```python
from build123d import *

# Parameters (mm, degrees)
SKETCH1_W           = 130
SKETCH1_H           = 98.5
SKETCH1_R           = 36.5
SKETCH1_R_2         = 5
BOSS_EXTRUDE1_DEPTH = 6
SKETCH2_W           = 130
SKETCH2_H           = 6
BOSS_EXTRUDE2_DEPTH = 75
CHAMFER1_SIZE       = 8
CUT_EXTRUDE1_DEPTH  = 7
BOSS_EXTRUDE3_START = -0.1
BOSS_EXTRUDE3_DEPTH = 3
BOSS_EXTRUDE4_START = -0.1
BOSS_EXTRUDE4_DEPTH = 3
FILLET1_R           = 2


with BuildPart() as part:
    # Sketch1 → Boss-Extrude1 (new body)
    with BuildSketch(Plane.XY):
        with Locations((-0.4, 43.207953426)):
            Rectangle(SKETCH1_W, SKETCH1_H)
        with Locations((-0.4, 45.807953426)):
            Circle(SKETCH1_R, mode=Mode.SUBTRACT)
        with Locations((-35.2, 80.607953426)):
            Circle(SKETCH1_R_2, mode=Mode.SUBTRACT)
        with Locations((34.4, 80.607953426)):
            Circle(SKETCH1_R_2, mode=Mode.SUBTRACT)
        with Locations((34.4, 11.007953426)):
            Circle(SKETCH1_R_2, mode=Mode.SUBTRACT)
        with Locations((-35.2, 11.007953426)):
            Circle(SKETCH1_R_2, mode=Mode.SUBTRACT)
    extrude(amount=BOSS_EXTRUDE1_DEPTH)

    # Sketch2 → Boss-Extrude2 (add)
    with BuildSketch(Plane.XY.offset(6)):
        with Locations((-0.4, -3.042046574)):
            Rectangle(SKETCH2_W, SKETCH2_H)
    extrude(amount=BOSS_EXTRUDE2_DEPTH)

    # Chamfer1
    chamfer1_edges = [part.edges().sort_by_distance(p)[0] for p in [
        (-65.4, -3.042046574, 81),
        (64.6, -3.042046574, 81),
        (-65.4, 92.457953426, 3),
        (64.6, 92.457953426, 3),
    ]]
    chamfer(chamfer1_edges, length=CHAMFER1_SIZE)

    # Sketch3 → Cut-Extrude1 (cut, through all)
    with BuildSketch(Plane(origin=(0, -0.042046574, 0), x_dir=(1, 0, 0), z_dir=(0, 1, 0))):
        with BuildLine():
            Line((-58.9, -68.5), (-58.9, -18.5))
            ThreePointArc((-58.9, -18.5), (-55.4, -15), (-51.9, -18.5))
            Line((-51.9, -18.5), (-51.9, -68.5))
            ThreePointArc((-51.9, -68.5), (-55.4, -72), (-58.9, -68.5))
        make_face()
        with BuildLine():
            Line((58.1, -68.5), (58.1, -18.5))
            ThreePointArc((58.1, -18.5), (54.6, -15), (51.1, -18.5))
            Line((51.1, -18.5), (51.1, -68.5))
            ThreePointArc((51.1, -68.5), (54.6, -72), (58.1, -68.5))
        make_face()
    extrude(amount=-CUT_EXTRUDE1_DEPTH, mode=Mode.SUBTRACT)

    # Sketch4 → Boss-Extrude3 (add)
    with BuildSketch(Plane.ZY.offset(65.4).offset(BOSS_EXTRUDE3_START)):
        Polygon((6, 37.957953426), (35, -0.042046574), (12.357101974, -0.042046574), (6, 8.287949116), align=None)
    extrude(amount=-BOSS_EXTRUDE3_DEPTH)

    # Sketch5 → Boss-Extrude4 (add)
    with BuildSketch(Plane(origin=(64.6, 0, 0), x_dir=(0, 0, -1), z_dir=(1, 0, 0)).offset(BOSS_EXTRUDE4_START)):
        Polygon((-6, 8.287949116), (-6, 37.957953426), (-35, -0.042046574), (-12.357101974, -0.042046574), align=None)
    extrude(amount=-BOSS_EXTRUDE4_DEPTH)

    # Fillet1
    fillet1_edges = [part.edges().sort_by_distance(p)[0] for p in [
        (-0.4, -0.042046574, 6),
        (-0.4, -6.042046574, 0),
    ]]
    fillet(fillet1_edges, radius=FILLET1_R)


solid = part.part
```
For this review, take the finished solid that the model builds, in its own axes (mm). A direction names the side the tool comes from. Round coordinates to 2 decimals unless told otherwise and drop trailing zeros. Order: outer loops, then holes, each group sorted by start corner. A loop starts at its lowest first (then second) coordinate and runs counter-clockwise, first axis right, second up.
Q1. We need section D-D, the plane x = -0.4. Give the boundary of the cut face in (y, z), plus the area to 3 significant figures.
Findings below:
outline: (-6.04, 2) arc R2 ccw to (-4.04, 0) - (9.31, 0) - (9.31, 6) - (1.96, 6) arc R2 cw to (-0.04, 8) - (-0.04, 81) - (-6.04, 81) - close; (82.31, 0) - (92.46, 0) - (92.46, 6) - (82.31, 6) - close
area: 603 mm2
Q2. Insertion check: P1, Ø2, axis at x = 20, z = 59, coming from the +Y side; P2, Ø6, axis at x = -51.5, y = 51, coming from the +Z side; P3, Ø8, axis at x = -27, y = 75.5, coming from the -Z side; P4, Ø14.5, axis at y = 10, z = 18, coming from the -X side. Each pin has a flat end and moves straight along its axis. Give the tip position at first contact, or say it passes through.
Findings below:
P1: stops at y = -0.04
P2: stops at z = 6
P3: stops at z = 0
P4: stops at x = -65.3
Q3. Wall thickness on line 1 (X direction, y = -0.5, z = 53); line 2 (Y direction, x = -0.4, z = 1.8); line 3 (X direction, y = 12.5, z = 21): over which ranges is each line inside the solid? List them lowest first.
Findings below:
line 1: x = -65.4 to -58.9, -51.9 to 51.1, 58.1 to 64.6
line 2: y = -6.03 to 9.31, 82.31 to 92.46
line 3: x = -65.3 to -62.3, 61.5 to 64.5
Q4. Mouldability with a two-part tool opening along Z and no side actions: class faces 1 (the flat face through (-61.3, -3.1, 77.1)), 2 (the cylindrical face through (33.316, 75.727, 2.958)), 3 (the flat face through (-63.821, 4.065, 9.223)) as pulls with the +Z half, pulls with the -Z half, needs draft (parallel to the pull), parting line crosses it, or undercut.
Findings below:
face 1: pulls with the +Z half
face 2: needs draft
face 3: undercut
Q5. We need section C-C, the plane y = 62. Give the boundary of the cut face in (x, z), plus the area to 3 significant figures.
Findings below:
outline: (-65.4, 0) - (-33.11, 0) - (-33.11, 6) - (-65.4, 6) - close; (32.31, 0) - (64.6, 0) - (64.6, 6) - (32.31, 6) - close
area: 387 mm2
Q6. We need section A-A, the plane x = -55.4. Give the boundary of the cut face in (y, z), plus the area to 3 significant figures.
Findings below:
outline: (-6.04, 2) arc R2 ccw to (-4.04, 0) - (92.46, 0) - (92.46, 6) - (1.96, 6) arc R2 cw to (-0.04, 8) - (-0.04, 15) - (-6.04, 15) - close; (-6.04, 72) - (-0.04, 72) - (-0.04, 81) - (-6.04, 81) - close
area: 699 mm2
Q7. We need section B-B, the plane z = 55. Give the boundary of the cut face in (x, y), plus the area to 3 significant figures.
Findings below:
outline: (-65.4, -6.04) - (-58.9, -6.04) - (-58.9, -0.04) - (-65.4, -0.04) - close; (-51.9, -6.04) - (51.1, -6.04) - (51.1, -0.04) - (-51.9, -0.04) - close; (58.1, -6.04) - (64.6, -6.04) - (64.6, -0.04) - (58.1, -0.04) - close
area: 696 mm2
Q8. Machinability: for faces 4 (the flat face through (61.5, 11, 14)), 5 (the flat face through (-58.9, -3, 44)), which of the approach directions +Z, -Z, +X, -X, +Y, -Y give a long, thin tool a straight path to every point of the face, cutting with its end or side? Answer none if there is none.
Findings below:
face 4: +Z, +Y
face 5: +Y, -Y
